Geometry check sheet. Reference: drawing and pictorial views, mm from the part's lowest x, y, z. Round coordinates to 2 decimals unless told otherwise and drop trailing zeros. Loops run counter-clockwise (first coordinate to the right, second up) from the corner with the lowest first, then second, coordinate; pieces in that order, holes last. Notation, with made-up numbers: (-8.5, -11) - (21.5, -11) arc R18 ccw to (21.5, 18) - close; hole circle Ø1 at (-26.5, -26.5). An arc over 180 degrees is marked (long way). Return JSON: item names as keys, results as strings.
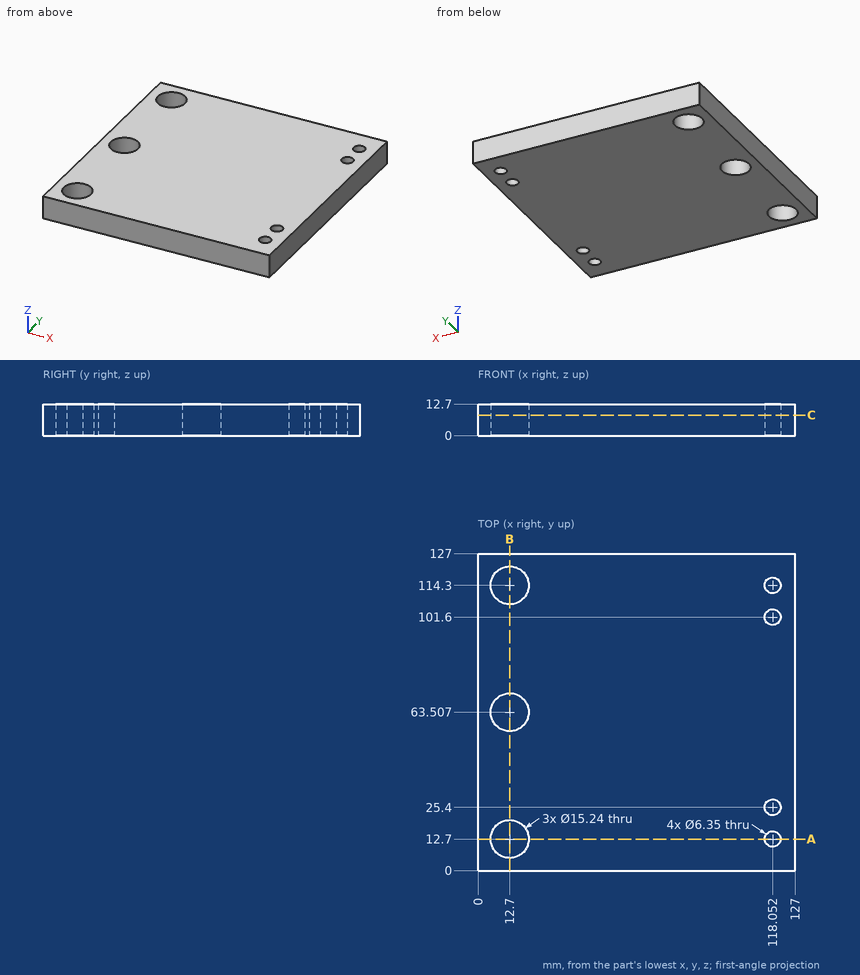
Q1. Scan lines: probe 1 along Y at (x, z) = (12.7, 4); probe 2 along Y at (x, z) = (19, 4) (1 decimal); probe 3 along X at (y, z) = (14.5, 6.25) (1 decimal). Record each from-to range of solid material in increasing order. Write a range as [from, to].
Answer key:
{"probe 1": "y = [0, 5.08], [20.32, 55.89], [71.13, 106.68], [121.92, 127]", "probe 2": "y = [0, 8.4], [17, 59.2], [67.8, 110], [118.6, 127]", "probe 3": "x = [0, 5.3], [20.1, 115.4], [120.7, 127]"}
Q2. Sectioned sample at B-B (x = 12.7). Enter the section's corners in (y, z), plus the area to 3 significant figures.
Answer key:
{"outline": "(0, 0) - (5.08, 0) - (5.08, 12.7) - (0, 12.7) - close; (20.32, 0) - (55.89, 0) - (55.89, 12.7) - (20.32, 12.7) - close; (71.13, 0) - (106.68, 0) - (106.68, 12.7) - (71.13, 12.7) - close; (121.92, 0) - (127, 0) - (127, 12.7) - (121.92, 12.7) - close", "area": "1,030 mm²"}
Q3. Sectioned sample at A-A (y = 12.7). Enter the section's corners in (x, z), plus the area to 3 significant figures.
Answer key:
{"outline": "(0, 0) - (5.08, 0) - (5.08, 12.7) - (0, 12.7) - close; (20.32, 0) - (114.88, 0) - (114.88, 12.7) - (20.32, 12.7) - close; (121.23, 0) - (127, 0) - (127, 12.7) - (121.23, 12.7) - close", "area": "1,340 mm²"}
Q4. Sectioned sample at C-C (z = 8.25). State how many separate pieces and enclosed holes the cut face has, plus the area to 3 significant figures.
Answer key:
{"separate pieces": "1", "enclosed holes": "7", "area": "15,500 mm²"}
